Could you check a few things on this drawing? It's one solid part, dimensions in mm from its lowest x, y, z. A direction names the side the tool comes from. Coordinates: 2 decimals unless noted, no trailing zeros. Write each loop counter-clockwise with the first axis right and the second up, starting at its lowest first coordinate (ties: lowest second). Pieces come first, ordered by that corner, then holes.
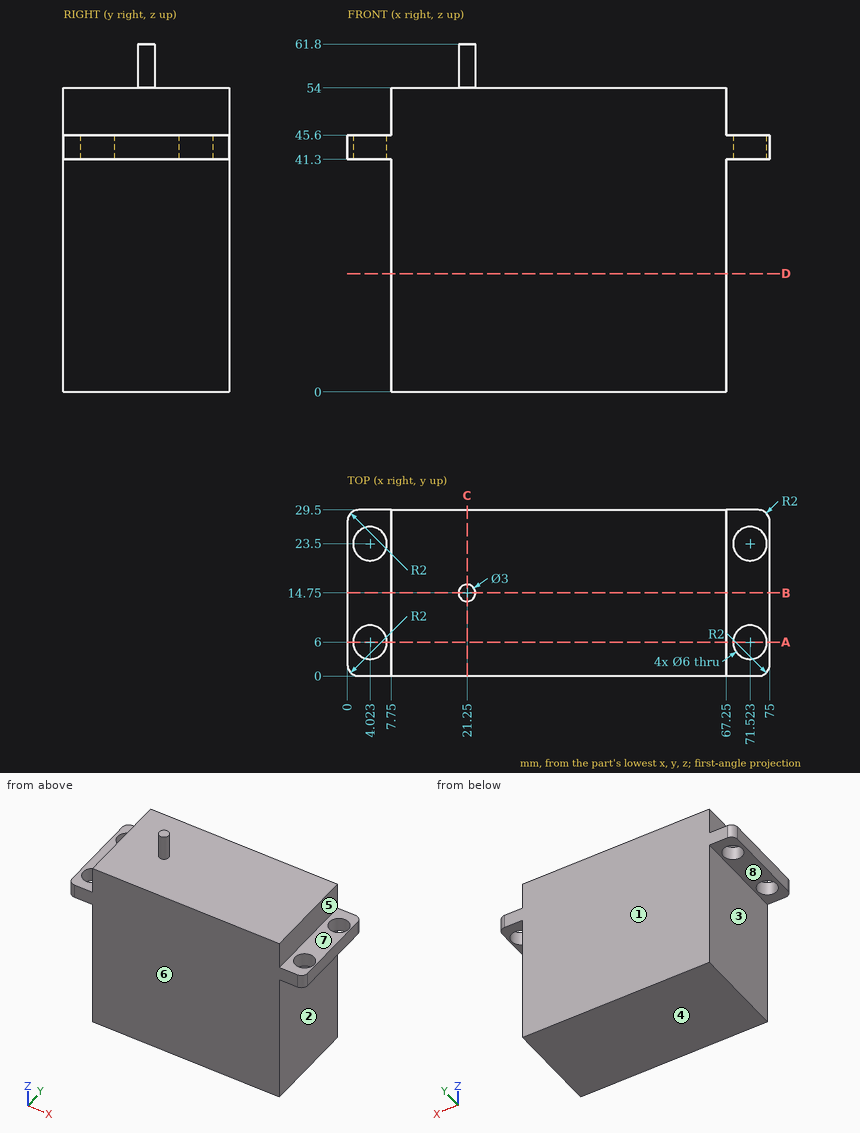
1) Imagine slicing it at C-C on x = 21.25. Please give me the cut outline in (y, z).
Values follow:
outline: (0, 0) - (29.5, 0) - (29.5, 54) - (16.25, 54) - (16.25, 61.8) - (13.25, 61.8) - (13.25, 54) - (0, 54) - close
2) Will these pins go through, and if not, where does the flat tip stop? pin 1 (5 mm diameter, centred on y = 15.5, z = 47, fed in from -X); pin 2 (2 mm diameter, centred on y = 15.5, z = 22, fed in from -X); pin 3 (2.5 mm diameter, centred on x = 3, y = 20, fed in from +Z); pin 4 (4 mm diameter, centred on y = 26.5, z = 33.5, fed in from +X).
Values follow:
pin 1: stops at x = 0
pin 2: stops at x = 7.75
pin 3: stops at z = 45.6
pin 4: stops at x = 67.25
3) On a 3-axis mill with a long thin cutter (end or side, diameter ignored), from which of +Z, -Z, +X, -X, +Y, -Y can I reach the whole of each face in a straight line? I mean the marked faces 1, 2, 3, 4 and 5. Say none if no direction works.
Values follow:
face 1: +Z, -Z, +X, -X, +Y
face 2: -Z, +X, +Y, -Y
face 3: -Z, -X, +Y, -Y
face 4: -Z, +X, -X, +Y, -Y
face 5: +Z, +X, +Y, -Y
4) Imagine slicing it at B-B on y = 14.75. Please give me the cut outline in (x, z), then the cut area to 3 significant figures.
Values follow:
outline: (0, 41.3) - (7.75, 41.3) - (7.75, 0) - (67.25, 0) - (67.25, 41.3) - (75, 41.3) - (75, 45.6) - (67.25, 45.6) - (67.25, 54) - (22.75, 54) - (22.75, 61.8) - (19.75, 61.8) - (19.75, 54) - (7.75, 54) - (7.75, 45.6) - (0, 45.6) - close
area: 3,300 mm2
5) We'd pull the mould along Z, two halves only. Please class the marked faces 6, 7 and 8: pulls with the +Z half, pulls with the -Z half, needs draft (parallel to the pull), parting line crosses it, or undercut.
Values follow:
face 6: needs draft
face 7: pulls with the +Z half
face 8: pulls with the -Z half
6) I need wall thicknesses on probe 1 along Z at (x, y) = (21, 16.5); probe 2 along X at (y, z) = (20.75, 13.5); probe 3 along Z at (x, y) = (68, 4.5). Which ranges of each line are inside material? Lowest first, please.
Values follow:
probe 1: z = 0 to 54
probe 2: x = 7.75 to 67.25
probe 3: z = 41.3 to 45.6
7) Imagine slicing it at D-D on z = 21. Please give me the cut outline in (x, y).
Values follow:
outline: (7.75, 0) - (67.25, 0) - (67.25, 29.5) - (7.75, 29.5) - close
8) Imagine slicing it at A-A on y = 6. Please give me the cut outline in (x, z), then the cut area to 3 significant figures.
Values follow:
outline: (0, 41.3) - (1.02, 41.3) - (1.02, 45.6) - (0, 45.6) - close; (7.02, 41.3) - (7.75, 41.3) - (7.75, 0) - (67.25, 0) - (67.25, 41.3) - (68.52, 41.3) - (68.52, 45.6) - (67.25, 45.6) - (67.25, 54) - (7.75, 54) - (7.75, 45.6) - (7.02, 45.6) - close; (74.52, 41.3) - (75, 41.3) - (75, 45.6) - (74.52, 45.6) - close
area: 3,230 mm2
